Could you check a few things on this model? Use its own coordinates, in mm. A direction names the side the tool comes from. Round coordinates to 2 decimals unless told otherwise and drop trailing zeros. Loops run counter-clockwise (first coordinate to the right, second up) from the corner with the lowest first, then second, coordinate; pieces in that order, holes last. Notation, with made-up numbers: M -1,26 L 34,26 A15 cw 34,54 Z; hole C -1.5,83.5 d2. An arc over 180 degrees is marked long. Answer in a Markdown table with one row per item.
```python
from build123d import *

# Parameters (mm, degrees)
SKETCH1_R           = 69.865875
SKETCH1_R_2         = 66.675
BOSS_EXTRUDE1_DEPTH = 2.54
BOSS_EXTRUDE2_START = -57.15
SKETCH2_R           = 73.025
SKETCH2_R_2         = 69.865875
BOSS_EXTRUDE2_DEPTH = 57.15
BOSS_EXTRUDE3_DEPTH = 6.35
FILLET2_R           = 12.7
SKETCH4_R           = 6.35
CUT_EXTRUDE1_DEPTH  = 0.254


with BuildPart() as part:
    # Sketch1 → Boss-Extrude1 (new body)
    with BuildSketch(Plane(origin=(0, 0, 0), x_dir=(1, 0, 0), z_dir=(0, 1, 0))):
        with Locations(Location((0, 0, 0), (0, 0, 270))):
            Circle(SKETCH1_R)
        with Locations(Location((0, 0, 0), (0, 0, 270))):
            Circle(SKETCH1_R_2, mode=Mode.SUBTRACT)
    extrude(amount=BOSS_EXTRUDE1_DEPTH)

    # Sketch2 → Boss-Extrude2 (add)
    with BuildSketch(Plane(origin=(0, 2.54, 0), x_dir=(1, 0, 0), z_dir=(0, 1, 0)).offset(BOSS_EXTRUDE2_START)):
        with Locations(Location((0, 0, 0), (0, 0, 270))):
            Circle(SKETCH2_R)
        with Locations(Location((0, 0, 0), (0, 0, 270))):
            Circle(SKETCH2_R_2, mode=Mode.SUBTRACT)
    extrude(amount=BOSS_EXTRUDE2_DEPTH)

    # Sketch3 → Boss-Extrude3 (add)
    with BuildSketch(Plane.XZ.offset(54.61)):
        with BuildLine():
            Line((-51.636472696, 51.636472696), (-51.636472696, 92.075))
            Line((-51.636472696, 92.075), (51.636472696, 92.075))
            Line((51.636472696, 92.075), (51.636472696, 51.636472696))
            ThreePointArc((51.636472696, 51.636472696), (0, 73.025), (-51.636472696, 51.636472696))
        make_face()
    extrude(amount=-BOSS_EXTRUDE3_DEPTH)

    # Fillet2
    fillet2_edges = [part.edges().sort_by_distance(p)[0] for p in [
        (51.636472696, -51.435, 51.636472696),
        (-51.636472696, -51.435, 51.636472696),
        (-51.636472696, -51.435, 92.075),
        (51.636472696, -51.435, 92.075),
    ]]
    fillet(fillet2_edges, radius=FILLET2_R)

    # Sketch4 → Cut-Extrude1 (cut)
    with BuildSketch(Plane(origin=(0, -48.26, 0), x_dir=(1, 0, 0), z_dir=(0, 1, 0))):
        with Locations(Location((-38.936472696, -79.375, 0), (0, 0, 270))):
            Circle(SKETCH4_R)
        with Locations(Location((38.936472696, -79.375, 0), (0, 0, 270))):
            Circle(SKETCH4_R)
    extrude(amount=-CUT_EXTRUDE1_DEPTH, mode=Mode.SUBTRACT)


solid = part.part
```
1) If we mould it in two halves opening along X, with no side actions, what happens to faces 4 (the face through (69.27, -27.69, -9.1)), 5 (the face through (-1, -51, 92.075)), 6 (the face through (51.636, -51, 68))? For each: released by +X, released by -X, zero draft, split by the parting line, or undercut.
Computed:
| item | result |
|---|---|
| face 4 | undercut |
| face 5 | zero draft |
| face 6 | released by +X |
2) Will these pins go through, and if not, where does the flat tip stop? P1, Ø6, axis at x = -53, y = -41.5, coming from the +Z side; P2, Ø10, axis at x = -42, z = 81, coming from the +Y side; P3, Ø11.5, axis at x = -38.94, z = 79.38, coming from the +Y side.
Computed:
| item | result |
|---|---|
| P1 | stops at z = 53.22 |
| P2 | stops at y = -48.26 |
| P3 | stops at y = -48.51 |
3) I want a section at A-A, the plane z = 0. Please give me the cut outline in (x, y) (3 decimals), plus the area to 3 significant figures.
Computed:
| item | result |
|---|---|
| outline | M -73.025,-54.61 L -69.866,-54.61 L -69.866,0 L -66.675,0 L -66.675,2.54 L -73.025,2.54 Z; M 66.675,0 L 69.866,0 L 69.866,-54.61 L 73.025,-54.61 L 73.025,2.54 L 66.675,2.54 Z |
| area | 377 mm² |
4) I want a section at D-D, the plane z = -36.5. Please give me the cut outline in (x, y).
Computed:
| item | result |
|---|---|
| outline | M -63.25,-54.61 L -59.57,-54.61 L -59.57,0 L -55.8,0 L -55.8,2.54 L -63.25,2.54 Z; M 55.8,0 L 59.57,0 L 59.57,-54.61 L 63.25,-54.61 L 63.25,2.54 L 55.8,2.54 Z |
5) Which directions (+Z, -Z, +X, -X, +Y, -Y) give clear straight access to the entire face, cutting with the end or side of a thin tool? Please do faces 1 (the face through (-51.636, -51, 68)), 2 (the face through (1, -48.26, 75)), 3 (the face through (-39, -48.514, 79)).
Computed:
| item | result |
|---|---|
| face 1 | +Z, -X, +Y, -Y |
| face 2 | +Z, +Y |
| face 3 | +Y |
6) I need wall thicknesses on line 1 (X direction, y = -8, z = -1.5); line 2 (X direction, y = -41.5, z = 0) (3 decimals); line 3 (Z direction, x = 7.5, y = -32). Which ranges of each line are inside material? Lowest first, please.
Computed:
| item | result |
|---|---|
| line 1 | x = -73.01 to -69.85, 69.85 to 73.01 |
| line 2 | x = -73.025 to -69.866, 69.866 to 73.025 |
| line 3 | z = -72.64 to -69.46, 69.46 to 72.64 |
7) I want a section at B-B, the plane x = 0. Please give me the cut outline in (y, z) (3 decimals).
Computed:
| item | result |
|---|---|
| outline | M -54.61,-73.025 L 2.54,-73.025 L 2.54,-66.675 L 0,-66.675 L 0,-69.866 L -54.61,-69.866 Z; M -54.61,69.866 L 0,69.866 L 0,66.675 L 2.54,66.675 L 2.54,73.025 L -48.26,73.025 L -48.26,92.075 L -54.61,92.075 Z |
8) I want a section at C-C, the plane y = -32.5. Please give me the cut outline in (x, z) (3 decimals).
Computed:
| item | result |
|---|---|
| outline | C 0,0 d146.05; hole C 0,0 d139.732 |
